Work out the finished part from the listing and answer in its coordinate system (mm). A direction names the side the tool comes from. Round coordinates to 2 decimals unless told otherwise and drop trailing zeros. Write each loop counter-clockwise with the first axis right and the second up, starting at its lowest first coordinate (ties: lowest second). Pieces come first, ordered by that corner, then holes. Notation, with made-up numbers: (50, 21) - (95, 21) arc R17 ccw to (95, 29) - close; hole circle Ø3 at (2.5, 41.5). An arc over 180 degrees is marked (long way). Write item = value, one per line. Start each with the question number.
from build123d import *

# Parameters (mm, degrees)
SKETCH1_W            = 37
SKETCH1_H            = 35
SKETCH1_R            = 2
BOSS_EXTRUDE1_DEPTH  = 3
SKETCH2_W            = 4
SKETCH2_H            = 35
BOSS_EXTRUDE2_DEPTH  = 30
SKETCH3_R            = 4
BOSS_EXTRUDE3_DEPTH  = 8
BOSS_EXTRUDE4_START  = 10
SKETCH4_R            = 4
BOSS_EXTRUDE4_DEPTH  = 10
BOSS_EXTRUDE5_DEPTH  = 4
MIRROR2_COPY_1_DEPTH = 4


with BuildPart() as part:
    # Sketch1 → Boss-Extrude1 (new body)
    with BuildSketch(Plane(origin=(0, 0, 0), x_dir=(1, 0, 0), z_dir=(0, 1, 0))):
        Rectangle(SKETCH1_W, SKETCH1_H)
        with Locations(Location((0, 0, 0), (0, 0, 270))):
            Circle(SKETCH1_R, mode=Mode.SUBTRACT)
    extrude(amount=BOSS_EXTRUDE1_DEPTH)

    # Sketch2 → Boss-Extrude2 (add)
    with BuildSketch(Plane(origin=(0, 3, 0), x_dir=(1, 0, 0), z_dir=(0, 1, 0))):
        with Locations((-16.5, 0)):
            Rectangle(SKETCH2_W, SKETCH2_H)
        with Locations((16.5, 0)):
            Rectangle(SKETCH2_W, SKETCH2_H)
    extrude(amount=BOSS_EXTRUDE2_DEPTH)

    # Sketch3 → Boss-Extrude3 (add)
    with BuildSketch(Plane.ZY.offset(18.5)):
        with Locations((0, 16.5)):
            Circle(SKETCH3_R)
    extrude(amount=BOSS_EXTRUDE3_DEPTH)

    # Sketch4 → Boss-Extrude4 (add)
    with BuildSketch(Plane(origin=(18.5, 0, 0), x_dir=(0, 0, -1), z_dir=(1, 0, 0)).offset(BOSS_EXTRUDE4_START)):
        with Locations(Location((0, 16.5, 0), (0, 0, 180))):
            Circle(SKETCH4_R)
    extrude(amount=-BOSS_EXTRUDE4_DEPTH)

    # Sketch5 → Boss-Extrude5 (add)
    with BuildSketch(Plane.XY.offset(17.5)):
        Polygon((-14.5, 10.979110478), (-6.272927794, 3), (-14.5, 3), align=None)
    boss_extrude5 = extrude(amount=-BOSS_EXTRUDE5_DEPTH)

    # Mirror1: Boss-Extrude5 across plane
    add(boss_extrude5.mirror(Plane(origin=(0, 0, 0), x_dir=(0, 0, 1), z_dir=(1, 0, 0))))

    # Mirror2: Boss-Extrude5 across plane
    add(boss_extrude5.mirror(Plane.XY))

    # Mirror2 copy 1 sketch → Mirror2 copy 1 (add)
    with BuildSketch(Plane(origin=(0, 0, -17.5), x_dir=(-1, 0, 0), z_dir=(0, 0, -1))):
        Polygon((-14.5, 10.979110478), (-6.272927794, 3), (-14.5, 3), align=None)
    extrude(amount=-MIRROR2_COPY_1_DEPTH)


solid = part.part
1. Find section D-D on y = 2. Give the vertices of the cut face in (x, z).
2. Consider line 1 (X direction, y = 29, z = -10.5); line 2 (X direction, y = 1.6, z = 0); line 3 (Z direction, x = -14, y = 6). Determine where each line is inside the solid, lowest interval first.
3. Find section B-B on x = 0. Give the vertices of the cut face in (y, z).
4. Which of the six approach directions +Z, -Z, +X, -X, +Y, -Y give full straight-line access (tool end or side, diameter ignored) to faces 4 (the face through (23.57, 12.534, -0.521)), 5 (the face through (-10.4, 7, -15.5)), 6 (the face through (-22.444, 20.466, -0.521)), 7 (the face through (0, 2, -17.5)), 8 (the face through (12, 5, -13.5))?
5. Find section C-C on z = 0. Give the vertices of the cut face in (x, y), plus the area to 3 significant figures.
6. Find section A-A on y = 27. Give the vertices of the cut face in (x, z), plus the area to 3 significant figures.
7. For a pull along Z with two mould halves and no side action, classify faces 1 (the face through (3, 3, 0)), 2 (the face through (10.4, 7, -15.5)), 3 (the face through (0, 2, 17.5)) as released by +Z, released by -Z, zero draft, split by the parting line, or undercut.
8. Each of these flat-tipped pins is pushed along its axis until it touches: pin 1 (3 mm diameter, centred on y = 11.5, z = -10, fed in from +X); pin 2 (2 mm diameter, centred on y = 6.5, z = 9, fed in from -X); pin 3 (3 mm diameter, centred on x = 22, y = 18, fed in from -Z). Where does it stop, or does it pass through?
Answer key:
q1.outline = (-18.5, -17.5) - (18.5, -17.5) - (18.5, 17.5) - (-18.5, 17.5) - close; hole circle Ø4 at (0, 0)
q2.line_1 = -18.5 to -14.5, 14.5 to 18.5
q2.line_2 = -18.5 to -2, 2 to 18.5
q2.line_3 = -17.5 to -13.5, 13.5 to 17.5
q3.outline = (0, -17.5) - (3, -17.5) - (3, -2) - (0, -2) - close; (0, 2) - (3, 2) - (3, 17.5) - (0, 17.5) - close
q4.face_4 = +X
q4.face_5 = +Z, -Z, +Y
q4.face_6 = -X
q4.face_7 = -Z, +X, -X, +Y, -Y
q4.face_8 = +Y
q5.outline = (-26.5, 12.5) - (-18.5, 12.5) - (-18.5, 0) - (-2, 0) - (-2, 3) - (-14.5, 3) - (-14.5, 33) - (-18.5, 33) - (-18.5, 20.5) - (-26.5, 20.5) - close; (2, 0) - (18.5, 0) - (18.5, 12.5) - (28.5, 12.5) - (28.5, 20.5) - (18.5, 20.5) - (18.5, 33) - (14.5, 33) - (14.5, 3) - (2, 3) - close
q5.area = 483 mm²
q6.outline = (-18.5, -17.5) - (-14.5, -17.5) - (-14.5, 17.5) - (-18.5, 17.5) - close; (14.5, -17.5) - (18.5, -17.5) - (18.5, 17.5) - (14.5, 17.5) - close
q6.area = 280 mm²
q7.face_1 = undercut
q7.face_2 = zero draft
q7.face_3 = released by +Z
q8.pin_1 = 18.5
q8.pin_2 = -18.5
q8.pin_3 = -4
